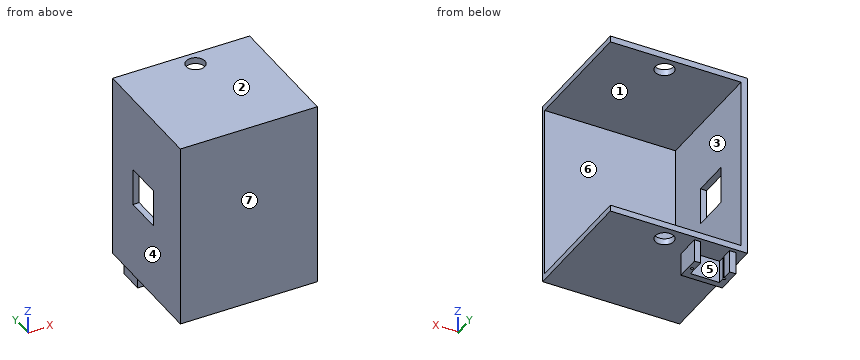
from build123d import *

# Parameters (mm, degrees)
COLLECTORSIZE_W         = 110
COLLECTORSIZE_H         = 150
BOSS_EXTRUDE1_DEPTH     = 200
COLLECTORSHAPE_W        = 110
COLLECTORSHAPE_H        = 100
CUT_EXTRUDE1_DEPTH      = 289.064276605
COLLECTORWALLS_W        = 129.645083566
COLLECTORWALLS_H        = 140
CUT_EXTRUDE2_DEPTH      = 97
CUT_EXTRUDE5_DEPTH      = 231.176079244
CUT_EXTRUDE5_DEPTH_BACK = 231.176079244
SKETCH1_R               = 7.5
BOSS_EXTRUDE3_DEPTH     = 18.25
SKETCH4_R               = 1.083059031
SKETCH4_R_2             = 1
CUT_EXTRUDE6_DEPTH      = 18.25
SKETCH2_2_W             = 30
SKETCH2_2_H             = 30
CUT_EXTRUDE7_DEPTH      = 10


with BuildPart() as part:
    # CollectorSize → Boss-Extrude1 (new body)
    with BuildSketch(Plane(origin=(0, 0, 0), x_dir=(1, 0, 0), z_dir=(0, 1, 0))):
        with Locations((88.111940299, -4.391791045)):
            Rectangle(COLLECTORSIZE_W, COLLECTORSIZE_H)
    extrude(amount=BOSS_EXTRUDE1_DEPTH)

    # CollectorShape → Cut-Extrude1 (cut, through all)
    with BuildSketch(Plane.XY.offset(79.391791045)):
        with Locations((88.111940299, 150)):
            Rectangle(COLLECTORSHAPE_W, COLLECTORSHAPE_H)
    extrude(amount=-CUT_EXTRUDE1_DEPTH, mode=Mode.SUBTRACT)

    # CollectorWalls → Cut-Extrude2 (cut)
    with BuildSketch(Plane(origin=(0, 100, 0), x_dir=(1, 0, 0), z_dir=(0, 1, 0))):
        with Locations((102.934482082, -4.391791045)):
            Rectangle(COLLECTORWALLS_W, COLLECTORWALLS_H)
    extrude(amount=-CUT_EXTRUDE2_DEPTH, mode=Mode.SUBTRACT)

    # Sketch1 → Cut-Extrude5 (cut, two sides: drawn at the far end of the back side and taken through both)
    with BuildSketch(Plane.XY.offset(79.391791045).offset(-CUT_EXTRUDE5_DEPTH_BACK)):
        with Locations((93.111940299, 88)):
            Circle(SKETCH1_R)
    extrude(amount=CUT_EXTRUDE5_DEPTH + CUT_EXTRUDE5_DEPTH_BACK, mode=Mode.SUBTRACT)

    # Sketch3 → Boss-Extrude3 (add)
    with BuildSketch(Plane(origin=(0, 0, -70.608208955), x_dir=(-1, 0, 0), z_dir=(0, 0, -1))):
        Polygon((-45.669947857, 81.9), (-68.919947857, 81.9), (-68.919947857, 96.9), (-73.919947857, 96.9), (-73.919947857, 76.9), (-40.669947857, 76.9), (-40.669947857, 96.9), (-45.669947857, 96.9), align=None)
    extrude(amount=BOSS_EXTRUDE3_DEPTH)

    # Sketch4 → Cut-Extrude6 (cut)
    with BuildSketch(Plane(origin=(0, 0, -88.858208955), x_dir=(-1, 0, 0), z_dir=(0, 0, -1))):
        with Locations((-44.876021334, 87.650563986)):
            Circle(SKETCH4_R)
        with Locations((-70.994947857, 88)):
            Circle(SKETCH4_R_2)
    extrude(amount=-CUT_EXTRUDE6_DEPTH, mode=Mode.SUBTRACT)

    # Sketch2<2> → Cut-Extrude7 (cut)
    with BuildSketch(Plane.ZY.offset(-33.111940299)):
        with Locations((4.391791045, 55)):
            Rectangle(SKETCH2_2_W, SKETCH2_2_H)
    extrude(amount=-CUT_EXTRUDE7_DEPTH, mode=Mode.SUBTRACT)


solid = part.part
Input: part model. Units: mm. Frame: model coordinates. Face numbers are marked on the shaded views. A direction names the side the tool comes from. Coordinates: 2 decimals unless noted, no trailing zeros. Loops run counter-clockwise (first coordinate to the right, second up) from the corner with the lowest first, then second, coordinate; pieces in that order, holes last. Notation, with made-up numbers: (87.5, 38.5) -> (105.5, 38.5) arc R18 cw to (105.5, 62.5) -> close; hole circle Ø6 at (74, 0.25). An arc over 180 degrees is marked (long way). One line per item, written item: value.
(1) Draft query along Z for the marked faces 1, 2, 3 and 4. Return one class per face: pulls with the +Z half, pulls with the -Z half, needs draft (parallel to the pull), parting line crosses it, or undercut.
Answer below:
face 1: undercut
face 2: pulls with the +Z half
face 3: undercut
face 4: needs draft
(2) Cut plane D-D (y = 93.5). Output: boundary loops of the cut face in (x, z).
Answer below:
outline: (33.11, -70.61) -> (40.67, -70.61) -> (40.67, -88.86) -> (45.67, -88.86) -> (45.67, -70.61) -> (68.92, -70.61) -> (68.92, -88.86) -> (73.92, -88.86) -> (73.92, -70.61) -> (88.01, -70.61) -> (88.01, -65.61) -> (38.11, -65.61) -> (38.11, 74.39) -> (88.01, 74.39) -> (88.01, 79.39) -> (33.11, 79.39) -> close; (98.21, -70.61) -> (143.11, -70.61) -> (143.11, -65.61) -> (98.21, -65.61) -> close; (98.21, 74.39) -> (143.11, 74.39) -> (143.11, 79.39) -> (98.21, 79.39) -> close
(3) Pin query (flat end, axial travel): pin 1 Ø4.5 at (y, z) = (89.5, -77.5) entering from -X; pin 2 Ø12 at (x, y) = (93.11, 88) entering from -Z; pin 3 Ø7 at (y, z) = (91, -78.5) entering from +X; pin 4 Ø10 at (x, z) = (63.5, -9.5) entering from +Y. Return the tip coordinate at first contact, or that it passes through.
Answer below:
pin 1: stops at x = 40.67
pin 2: passes through
pin 3: stops at x = 73.92
pin 4: stops at y = 3
(4) Cut plane B-B (x = 97). Output: boundary loops of the cut face in (y, z).
Answer below:
outline: (0, -70.61) -> (81.59, -70.61) -> (81.59, -65.61) -> (3, -65.61) -> (3, 74.39) -> (81.59, 74.39) -> (81.59, 79.39) -> (0, 79.39) -> close; (94.41, -70.61) -> (100, -70.61) -> (100, -65.61) -> (94.41, -65.61) -> close; (94.41, 74.39) -> (100, 74.39) -> (100, 79.39) -> (94.41, 79.39) -> close
(5) Cut plane C-C (z = -75). Output: boundary loops of the cut face in (x, y).
Answer below:
outline: (40.67, 76.9) -> (73.92, 76.9) -> (73.92, 96.9) -> (68.92, 96.9) -> (68.92, 81.9) -> (45.67, 81.9) -> (45.67, 86.91) arc R1.08 cw (long way) to (45.67, 88.39) -> (45.67, 96.9) -> (40.67, 96.9) -> close; hole circle Ø2 at (70.99, 88)
(6) Set-up query: the marked faces 5, 6 and 7. Return all of +Z, -Z, +X, -X, +Y, -Y with unobstructed straight access to the full face (end or side cutting, diameter ignored); none if empty.
Answer below:
face 5: -Z, +Y
face 6: +X, +Y
face 7: +Z, -Z, +X, -X, -Y
(7) Ray query, line 1 along Z through (x, y) = (94, 47.5); line 2 along Y through (x, z) = (75.5, -48); line 3 along X through (y, z) = (88, -69.6). Return the intervals inside material, ascending.
Answer below:
line 1: z = -70.61 to -65.61, 74.39 to 79.39
line 2: y = 0 to 3
line 3: x = 33.11 to 85.61, 100.61 to 143.11
(8) Cut plane A-A (z = 9.5). Output: boundary loops of the cut face in (x, y).
Answer below:
outline: (33.11, 0) -> (143.11, 0) -> (143.11, 3) -> (38.11, 3) -> (38.11, 40) -> (33.11, 40) -> close; (33.11, 70) -> (38.11, 70) -> (38.11, 100) -> (33.11, 100) -> close
